from build123d import *

# Parameters (mm, degrees)
SKETCH_1_W          = 9.55
SKETCH_1_H          = 16
EXTRUDE_1_DEPTH     = 17
SKETCH_2_W          = 8.05
SKETCH_2_H          = 16
CUT_EXTRUDE_1_DEPTH = 6.5
SKETCH_5_W          = 8.05
SKETCH_5_H          = 8.5
CUT_EXTRUDE_4_DEPTH = 2.8
SKETCH_6_W          = 8.05
SKETCH_6_H          = 2
CUT_EXTRUDE_5_DEPTH = 1.5
DRAFT_1_ANGLE       = 1
SKETCH_7_W          = 8.05
SKETCH_7_H          = 13.366556364
CUT_EXTRUDE_6_DEPTH = 1
FILLET_1_R          = 1.5
SKETCH_8_W          = 8.05
SKETCH_8_H          = 9
EXTRUDE_1747_DEPTH  = 1.5
SKETCH_9_R          = 0.6
EXTRUDE_3_DEPTH     = 10
FILLET_2_R          = 1.5
SKETCH_10_W         = 7.5
SKETCH_10_H         = 7.5
EXTRUDE_4_DEPTH     = 1.2
FILLET_4_R          = 0.5


with BuildPart() as part:
    # 草图1 → 拉伸1 (new body)
    with BuildSketch(Plane(origin=(0, 0, 0), x_dir=(1, 0, 0), z_dir=(0, 1, 0))):
        Rectangle(SKETCH_1_W, SKETCH_1_H)
    extrude(amount=EXTRUDE_1_DEPTH)

    # 草图2 → 切除-拉伸1 (cut)
    with BuildSketch(Plane(origin=(0, 17, 0), x_dir=(-1, 0, 0), z_dir=(0, 1, 0))):
        Rectangle(SKETCH_2_W, SKETCH_2_H)
    extrude(amount=-CUT_EXTRUDE_1_DEPTH, mode=Mode.SUBTRACT)

    # 草图5 → 切除-拉伸4 (cut)
    with BuildSketch(Plane(origin=(0, 0, -8), x_dir=(-1, 0, 0), z_dir=(0, 0, -1))):
        with Locations((0, 6.25)):
            Rectangle(SKETCH_5_W, SKETCH_5_H)
    cut_extrude_4 = extrude(amount=-CUT_EXTRUDE_4_DEPTH, mode=Mode.SUBTRACT)

    # 草图6 → 切除-拉伸5 (cut)
    with BuildSketch(Plane(origin=(0, 0, -8), x_dir=(-1, 0, 0), z_dir=(0, 0, -1))):
        with Locations((0, 1)):
            Rectangle(SKETCH_6_W, SKETCH_6_H)
    cut_extrude_5 = extrude(amount=-CUT_EXTRUDE_5_DEPTH, mode=Mode.SUBTRACT)

    # 镜向3: 切除-拉伸4, 切除-拉伸5 across plane
    add(cut_extrude_4.mirror(Plane.XY), mode=Mode.SUBTRACT)
    add(cut_extrude_5.mirror(Plane.XY), mode=Mode.SUBTRACT)

    # 拔模1
    draft_1_faces = [part.faces().sort_by_distance(p)[0] for p in [
        (4.4, 8.5, 8),
        (-4.4, 8.5, 8),
        (0, 1, 6.5),
        (0, 6.25, 5.2),
        (0, 1, -6.5),
        (-4.4, 8.5, -8),
        (0, 6.25, -5.2),
        (4.4, 8.5, -8),
    ]]
    draft(draft_1_faces, Plane(origin=(4.025, 10.5, -8), x_dir=(0, 0, 1), z_dir=(0, 1, 0)), DRAFT_1_ANGLE)

    # 草图7 → 切除-拉伸6 (cut)
    with BuildSketch(Plane.XZ):
        Rectangle(SKETCH_7_W, SKETCH_7_H)
    extrude(amount=-CUT_EXTRUDE_6_DEPTH, mode=Mode.SUBTRACT)

    # 圆角1
    fillet_1_edges = [part.edges().sort_by_distance(p)[0] for p in [
        (4.4, 17, -7.886542078),
        (4.4, 17, 7.886542078),
        (-4.4, 17, -7.886542078),
        (-4.4, 17, 7.886542078),
    ]]
    fillet(fillet_1_edges, radius=FILLET_1_R)

    # 草图8 → Extrude 1747 (add)
    with BuildSketch(Plane(origin=(0, 10.5, 0), x_dir=(-1, 0, 0), z_dir=(0, 1, 0))):
        Rectangle(SKETCH_8_W, SKETCH_8_H)
    extrude(amount=EXTRUDE_1747_DEPTH)

    # 草图9 → 拉伸3 (add)
    with BuildSketch(Plane.XZ.offset(-1)):
        with Locations(Location((0, 0, 0), (0, 0, 90))):
            Circle(SKETCH_9_R)
    extrude(amount=EXTRUDE_3_DEPTH)

    # 圆角2
    fillet_2_edges = [part.edges().sort_by_distance(p)[0] for p in [
        (0, 12, -4.5),
        (0, 12, 4.5),
    ]]
    fillet(fillet_2_edges, radius=FILLET_2_R - 0.0001)  # a hair under: the kernel refuses the full size

    # 草图10 → 拉伸4 (add)
    with BuildSketch(Plane(origin=(0, 12, 0), x_dir=(-1, 0, 0), z_dir=(0, 1, 0))):
        Rectangle(SKETCH_10_W, SKETCH_10_H)
    extrude(amount=EXTRUDE_4_DEPTH)

    # 圆角4
    fillet_4_edges = [part.edges().sort_by_distance(p)[0] for p in [
        (3.75, 13.2, 0),
        (0, 13.2, -3.75),
        (-3.75, 13.2, 0),
        (0, 13.2, 3.75),
    ]]
    fillet(fillet_4_edges, radius=FILLET_4_R)


solid = part.part
The model under review builds one solid part; all positions refer to its coordinate system, in mm. A direction names the side the tool comes from. Round coordinates to 2 decimals unless told otherwise and drop trailing zeros. Write each loop counter-clockwise with the first axis right and the second up, starting at its lowest first coordinate (ties: lowest second). Pieces come first, ordered by that corner, then holes. Notation, with made-up numbers: (65, 0.5) -> (74, 0.5) arc R14 ccw to (74, 21.5) -> close; hole circle Ø11 at (8.5, -37). An arc over 180 degrees is marked (long way). Answer as a JSON object with one key per item and string values.
1. To check wall thickness, follow line 1 along X through (y, z) = (6.25, -7.25) (3 decimals); line 2 along Y through (x, z) = (-2, 0.25); line 3 along Z through (x, y) = (-3, 9). State the ranges of each line that lie inside material, in increasing order.
Results found:
{"line 1": "x = -4.775 to -4.025, 4.025 to 4.775", "line 2": "y = 1 to 13.2", "line 3": "z = -5.23 to 5.23"}
2. Machinability: for faces 1 (the face through (-0.506, -3.93, 0.323)), 2 (the face through (-4.025, 12.2, 0.1)), 3 (the face through (0, 2, 6)), 4 (the face through (0, 2, -6)), which of the approach directions +Z, -Z, +X, -X, +Y, -Y give a long, thin tool a straight path to every point of the face, cutting with its end or side? Answer none if there is none.
Results found:
{"face 1": "-Y", "face 2": "none", "face 3": "+Z, +Y", "face 4": "-Z, +Y"}
3. We need section B-B on z = 2. State the section outline as (x, y) points (3 decimals).
Results found:
{"outline": "(-4.775, 0) -> (-4.025, 0) -> (-4.025, 1) -> (4.025, 1) -> (4.025, 0) -> (4.775, 0) -> (4.775, 17) -> (4.025, 17) -> (4.025, 12) -> (3.75, 12) -> (3.75, 12.7) arc R0.5 ccw to (3.25, 13.2) -> (-3.25, 13.2) arc R0.5 ccw to (-3.75, 12.7) -> (-3.75, 12) -> (-4.025, 12) -> (-4.025, 17) -> (-4.775, 17) -> close"}
4. We need section D-D on z = 0. State the section outline as (x, y) points (3 decimals).
Results found:
{"outline": "(-4.775, 0) -> (-4.025, 0) -> (-4.025, 1) -> (-0.6, 1) -> (-0.6, -9) -> (0.6, -9) -> (0.6, 1) -> (4.025, 1) -> (4.025, 0) -> (4.775, 0) -> (4.775, 17) -> (4.025, 17) -> (4.025, 12) -> (3.75, 12) -> (3.75, 12.7) arc R0.5 ccw to (3.25, 13.2) -> (-3.25, 13.2) arc R0.5 ccw to (-3.75, 12.7) -> (-3.75, 12) -> (-4.025, 12) -> (-4.025, 17) -> (-4.775, 17) -> close"}
5. We need section C-C on y = 7.25. State the section outline as (x, z) points (3 decimals).
Results found:
{"outline": "(-4.775, -8.057) -> (-4.025, -8.057) -> (-4.025, -5.257) -> (4.025, -5.257) -> (4.025, -8.057) -> (4.775, -8.057) -> (4.775, 8.057) -> (4.025, 8.057) -> (4.025, 5.257) -> (-4.025, 5.257) -> (-4.025, 8.057) -> (-4.775, 8.057) -> close"}
6. Clearance check with flat-ended pins moving along their axes: pin 1 (1 mm diameter, centred on x = 3, y = 1.5, fed in from -Z); pin 2 (1 mm diameter, centred on x = 2, z = 4.5, fed in from +Y); pin 3 (1.5 mm diameter, centred on x = -2, z = 4, fed in from +Y). State where each tip first meets the part, or that it passes through.
Results found:
{"pin 1": "stops at z = -6.67", "pin 2": "stops at y = 11.62", "pin 3": "stops at y = 13.2"}
